Work out the finished part from the listing and answer in its coordinate system (mm). A direction names the side the tool comes from. Coordinates: 2 decimals unless noted, no trailing zeros. Order: outer loops, then holes, each group sorted by start corner. A loop starts at its lowest first (then second) coordinate and runs counter-clockwise, first axis right, second up. Notation, with made-up numbers: (80.5, 60) -> (91.5, 60) arc R31 ccw to (91.5, 97) -> close; hole circle Ø7 at (22, 21). An arc over 180 degrees is marked (long way). Write item = value, one per line. Start each with the question number.
Q1. Flat-ended cylindrical pins translate along their axes: pin 1 (5 mm diameter, centred on y = 15, z = 11.5, fed in from +X); pin 2 (4 mm diameter, centred on x = 17.5, y = 17, fed in from +Z); pin 3 (7.5 mm diameter, centred on x = 6, z = 20.5, fed in from -Y). Find the tip coordinate at first contact, or state that the pin passes through.
Q2. Straight lines are drawn through the part: L1, parallel to Y at x = -9, z = 21.5; L2, parallel to Z at x = -16, y = -17; L3, parallel to X at y = 16, z = 28.5. For each, find the intervals that lie inside material, in ascending order. Write a range as from..to.
Q3. The part is cut by section A-A, the plane x = -15. Determine the outline of the cut face in (y, z).
Q4. Which of the six approach directions +Z, -Z, +X, -X, +Y, -Y give full straight-line access (tool end or side, diameter ignored) to faces 1 (the flat face through (2, -2, 5)), 2 (the flat face through (25, 0, 1))?
Q5. The part is cut by section B-B, the plane y = 9. Determine the outline of the cut face in (x, z), plus the area to 3 significant figures.
```python
from build123d import *

# Parameters (mm, degrees)
F0_W      = 50
F0_H      = 50
F1_DEPTH  = 5
F2_W      = 50
F2_H      = 5
F3_DEPTH  = 25
F4_W      = 5
F4_H      = 45
F5_DEPTH  = 25
F7_DEPTH  = 5
F9_DEPTH  = 5
F10_W     = 50
F10_H     = 50
F11_DEPTH = 5


with BuildPart() as f1:
    # F0 (on Top) → F1 (new body)
    with BuildSketch(Plane.XY):
        Rectangle(F0_W, F0_H)
    extrude(amount=F1_DEPTH)

    # F2 (on face) → F3 (join)
    with BuildSketch(Plane.XY.offset(5)):
        with Locations((0, 22.5)):
            Rectangle(F2_W, F2_H)
    extrude(amount=F3_DEPTH)

    # F4 (on face) → F5 (join)
    with BuildSketch(Plane.XY.offset(5)):
        with Locations((-22.5, -2.5)):
            Rectangle(F4_W, F4_H)
    extrude(amount=F5_DEPTH)

    # F6 (on face) → F7 (cut)
    with BuildSketch(Plane(origin=(0, 25, 0), x_dir=(-1, 0, 0), z_dir=(0, 1, 0))):
        Polygon((-25, 30), (-25, 17), (8, 30), align=None)
    extrude(amount=-F7_DEPTH, mode=Mode.SUBTRACT)

    # F8 (on face) → F9 (cut)
    with BuildSketch(Plane(origin=(-25, 0, 0), x_dir=(0, -1, 0), z_dir=(-1, 0, 0))):
        Polygon((25, 30), (-8, 30), (25, 17), align=None)
    extrude(amount=-F9_DEPTH, mode=Mode.SUBTRACT)

    # F10 (on face) → F11 (join)
    with BuildSketch(Plane(origin=(0, 0, 0), x_dir=(1, 0, 0), z_dir=(0, 0, -1))):
        Rectangle(F10_W, F10_H)
    extrude(amount=F11_DEPTH)


solid = f1.part
```
Model answer:
q1.pin_1 = -20
q1.pin_2 = 5
q1.pin_3 = 20
q2.L1 = 20..25
q2.L2 = -5..5
q2.L3 = -25..-20
q3.outline = (-25, -5) -> (25, -5) -> (25, 30) -> (20, 30) -> (20, 5) -> (-25, 5) -> close
q4.face_1 = +Z, +X, -Y
q4.face_2 = +Z, -Z, +X, +Y, -Y
q5.outline = (-25, -5) -> (25, -5) -> (25, 5) -> (-20, 5) -> (-20, 30) -> (-25, 30) -> close
q5.area = 625 mm2
